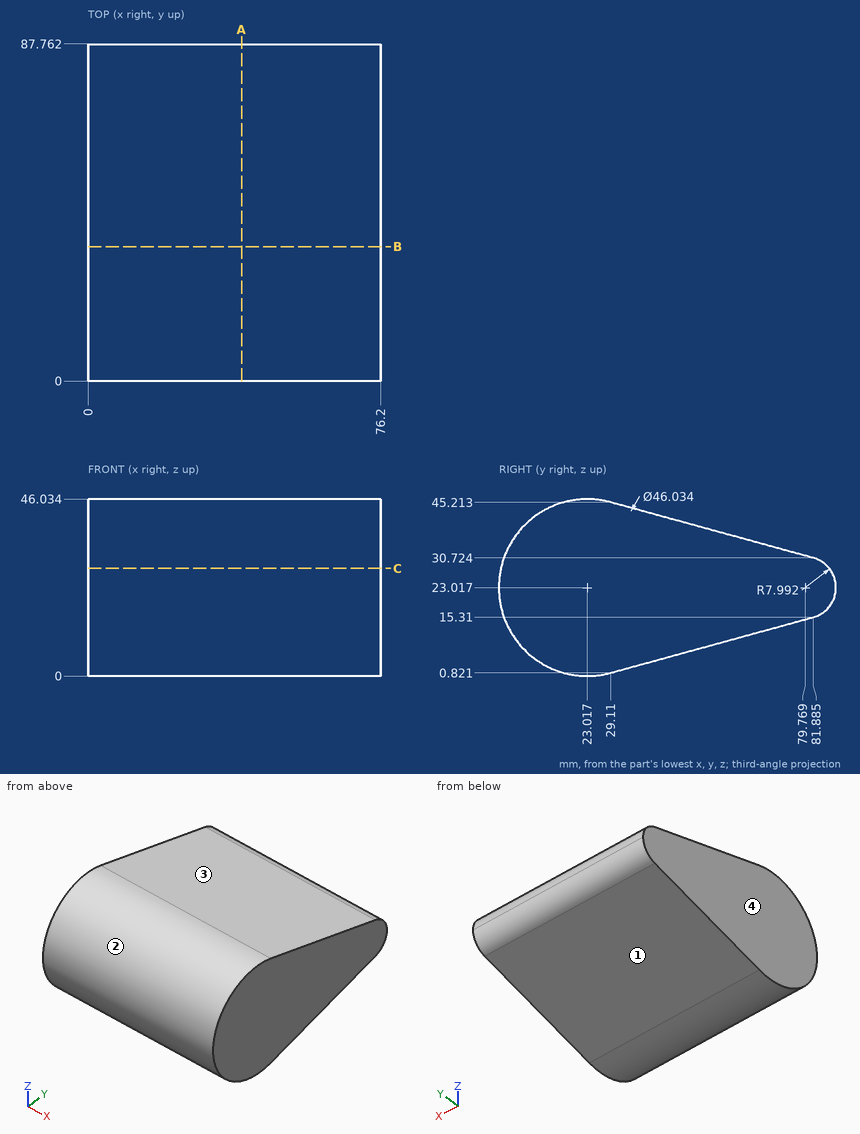
Can you work these out from the drawing? Everything is in mm from the part's minimum corner. Round coordinates to 2 decimals unless told otherwise and drop trailing zeros. Write each loop counter-clockwise with the first axis right and the second up, starting at its lowest first coordinate (ties: lowest second). Pieces come first, ordered by that corner, then holes. Notation, with made-up numbers: M 84.25,52.5 L 141.25,52.5 A37 ccw 141.25,88.5 Z; hole C -16.75,-36.5 d3. An arc over 180 degrees is marked long. Use a Markdown table: item, result.
Item 1: I want a section at A-A (x = 40). List the corners of the cut face in (y, z) for me (1 decimal).
Found:
| item | result |
|---|---|
| outline | M 29.1,0.8 L 81.9,15.3 A8 ccw 81.9,30.7 L 29.1,45.2 A23 ccw long Z |
Item 2: We'd pull the mould along Z, two halves only. Please class the marked faces 1, 2, 3 and 4: released by +Z, released by -Z, zero draft, split by the parting line, or undercut.
Found:
| item | result |
|---|---|
| face 1 | released by -Z |
| face 2 | split by the parting line |
| face 3 | released by +Z |
| face 4 | zero draft |
Item 3: If I drill on line 1 along Y through (x, z) = (54, 17); line 2 along Z through (x, y) = (15.5, 21) (1 decimal); line 3 along Z through (x, y) = (56, 63) (1 decimal), over which ranges is the centre line in solid material (lowest first)? Write a range as [from, to].
Found:
| item | result |
|---|---|
| line 1 | y = [0.8, 85.03] |
| line 2 | z = [0.1, 45.9] |
| line 3 | z = [10.1, 35.9] |
Item 4: For pin 1 Ø2 at (x, y) = (37.5, 56) entering from -Z; pin 2 Ø1 at (x, z) = (45.5, 32) entering from -Y; pin 3 Ø2 at (x, y) = (35, 59.5) entering from -Z, each with a flat end and sliding along its axis, tell me the tip position at first contact or that it passes through.
Found:
| item | result |
|---|---|
| pin 1 | stops at z = 7.93 |
| pin 2 | stops at y = 1.62 |
| pin 3 | stops at z = 8.89 |
Item 5: I want a section at B-B (y = 35). List the corners of the cut face in (x, z) for me (1 decimal), and give its area (3 significant figures).
Found:
| item | result |
|---|---|
| outline | M 0,2.4 L 76.2,2.4 L 76.2,43.6 L 0,43.6 Z |
| area | 3,140 mm2 |
Item 6: I want a section at C-C (z = 28). List the corners of the cut face in (x, y) for me (1 decimal), and give its area (3 significant figures).
Found:
| item | result |
|---|---|
| outline | M 0,0.5 L 76.2,0.5 L 76.2,86 L 0,86 Z |
| area | 6,510 mm2 |
